For this review, take the finished solid that the model builds, in its own axes (mm). Round coordinates to 2 decimals unless told otherwise and drop trailing zeros. Write each loop counter-clockwise with the first axis right and the second up, starting at its lowest first coordinate (ties: lowest second). Pieces come first, ordered by that corner, then holes. Notation, with made-up numbers: (10, 39.5) - (43, 39.5) arc R26 cw to (43, 73.5) - close; hole circle Ø11 at (-10, 12.5). An arc over 180 degrees is marked (long way). One line per item, written item: value. Start each with the question number.
Q1. For probe 1 along X at (y, z) = (1.2, -110); probe 2 along X at (y, z) = (1.4, -37); probe 3 along Z at (x, y) = (1.45, 0.25), list the stretches that pass through material, from the lowest coordinate up.
Q2. Clearance check with a flat-ended pin moving along its axis: pin 1 Ø2 at (x, z) = (-1.5, -85.5) entering from +Y. State where the tip first meets the part, or that it passes through.
Q3. Add section A-A on z = -138.5. Write out the cut boundary in (x, y), and give its area (3 significant figures).
Q4. Add section B-B on z = -189. Write out the cut boundary in (x, y), and give its area (3 significant figures).
```python
from build123d import *

# Parameters (mm, degrees)
F0_R      = 1
F1_DEPTH  = 180
F2_DEPTH  = 203.3524
F1_FACE_W = 2.8867513459
F1_FACE_H = 180


with BuildPart() as f1:
    # F0 (on Top) → F1 (new body)
    with BuildSketch(Plane.XY):
        with BuildLine():
            ThreePointArc((-1.3365232204, -2.1127483715), (-2.213837243, -1.1614321596), (-2.4979553725, 0.1010888571))
            Line((-2.4979553725, 0.1010888571), (-2.5563190236, -1.3411064025))
            Line((-2.5563190236, -1.3411064025), (-1.3365232204, -2.1127483715))
        make_face()
        with BuildLine():
            Line((-0.1167272981, -2.8843904159), (1.1614322324, -2.2138372048))
            ThreePointArc((1.1614322324, -2.2138372048), (-0.1010888301, -2.4979553736), (-1.3365232204, -2.1127483715))
            Line((-1.3365232204, -2.1127483715), (-0.1167272981, -2.8843904159))
        make_face()
        with BuildLine():
            ThreePointArc((-1.1614322324, 2.2138372048), (0.1010888127, 2.4979553743), (1.3365231909, 2.1127483902))
            Line((1.3365231909, 2.1127483902), (0.1167272981, 2.8843904159))
            Line((0.1167272981, 2.8843904159), (-1.1614322324, 2.2138372048))
        make_face()
        with BuildLine():
            ThreePointArc((-2.4979553725, 0.1010888571), (-2.112748401, 1.3365231738), (-1.1614322324, 2.2138372048))
            Line((-1.1614322324, 2.2138372048), (-2.4395917255, 1.5432840134))
            Line((-2.4395917255, 1.5432840134), (-2.4979553725, 0.1010888571))
        make_face()
        with BuildLine():
            Line((2.4395917255, -1.5432840134), (2.4979553754, -0.101088785))
            ThreePointArc((2.4979553754, -0.101088785), (2.1127484203, -1.3365231433), (1.1614322324, -2.2138372048))
            Line((1.1614322324, -2.2138372048), (2.4395917255, -1.5432840134))
        make_face()
        with BuildLine():
            ThreePointArc((1.3365231909, 2.1127483902), (2.1898981685, 1.2059626907), (2.5, 0))
            ThreePointArc((2.5, 0), (2.4994887916, -0.0505547301), (2.4979553754, -0.101088785))
            Line((2.4979553754, -0.101088785), (2.5563190236, 1.3411064025))
            Line((2.5563190236, 1.3411064025), (1.3365231909, 2.1127483902))
        make_face()
        with BuildLine():
            ThreePointArc((2.4979553754, -0.101088785), (2.4994887916, -0.0505547301), (2.5, 0))
            ThreePointArc((2.5, 0), (2.1898981685, 1.2059626907), (1.3365231909, 2.1127483902))
            ThreePointArc((1.3365231909, 2.1127483902), (0.1010888127, 2.4979553743), (-1.1614322324, 2.2138372048))
            ThreePointArc((-1.1614322324, 2.2138372048), (-2.112748401, 1.3365231738), (-2.4979553725, 0.1010888571))
            ThreePointArc((-2.4979553725, 0.1010888571), (-2.213837243, -1.1614321596), (-1.3365232204, -2.1127483715))
            ThreePointArc((-1.3365232204, -2.1127483715), (-0.1010888301, -2.4979553736), (1.1614322324, -2.2138372048))
            ThreePointArc((1.1614322324, -2.2138372048), (2.1127484203, -1.3365231433), (2.4979553754, -0.101088785))
        make_face()
        Circle(F0_R, mode=Mode.SUBTRACT)
    extrude(amount=-F1_DEPTH)

    # F0 (on Top) → F2 (join)
    with BuildSketch(Plane.XY):
        Circle(F0_R)
    extrude(amount=-F2_DEPTH)

    # F1_face (on face) → F5 section 0
    with BuildSketch(Plane(origin=(1.3365231609, 2.1127484092, -90), x_dir=(-0.8450993637, 0.5346092643, 0), z_dir=(0.5346092643, 0.8450993637, 0)), mode=Mode.PRIVATE) as f5_s0:
        Rectangle(F1_FACE_W, F1_FACE_H)
    loft([Vertex(0, 0, -200), f5_s0.sketch])


solid = f1.part
```
Result set:
1. probe 1: x = -2.45 to 2.55
1. probe 2: x = -2.45 to 2.46
1. probe 3: z = -180 to 0
2. pin 1: stops at y = 2.56
3. outline: (-2.56, -1.34) - (-0.12, -2.88) - (2.44, -1.54) - (2.56, 1.34) - (0.12, 2.88) - (-2.44, 1.54) - close
3. area: 21.7 mm^2
4. outline: (0.04, 1) arc R1 ccw (long way) to (0.89, 0.46) - (1.41, 0.74) - (0.06, 1.59) - close
4. area: 3.71 mm^2
